For this review, take the finished solid that the model builds, in its own axes (mm). Face numbers are marked on the shaded views. A direction names the side the tool comes from. Coordinates: 2 decimals unless noted, no trailing zeros. Write each loop counter-clockwise with the first axis right and the second up, starting at its lowest first coordinate (ties: lowest second). Pieces come first, ordered by that corner, then holes.
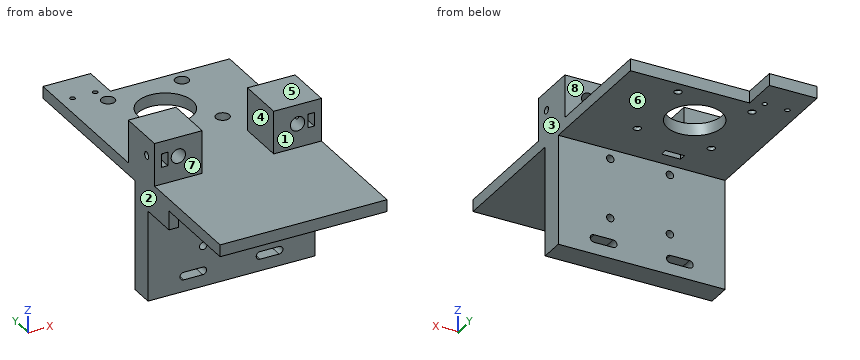
```python
from build123d import *

# Parameters (mm, degrees)
SKETCH1_W           = 70
SKETCH1_H           = 120
BOSS_EXTRUDE1_DEPTH = 5
SKETCH2_W           = 20
SKETCH2_H           = 20
BOSS_EXTRUDE2_DEPTH = 18
CUT_EXTRUDE1_REACH  = 83.572
SKETCH3_R           = 3
CUT_EXTRUDE2_REACH  = 75.171
SKETCH4_R           = 11.5
SKETCH4_R_2         = 1.55
SKETCH5_W           = 20
SKETCH5_H           = 15
SKETCH5_R           = 1.05
BOSS_EXTRUDE3_DEPTH = 5
SKETCH6_W           = 70
SKETCH6_H           = 10
BOSS_EXTRUDE4_DEPTH = 46
SKETCH7_W           = 2.6
SKETCH7_H           = 5.7
CUT_EXTRUDE3_DEPTH  = 10
SKETCH8_R           = 1.5
CUT_EXTRUDE4_DEPTH  = 8
CUT_EXTRUDE5_START  = -8
SKETCH9_R           = 1.5
CUT_EXTRUDE5_DEPTH  = 8
SKETCH10_R          = 2.85
CUT_EXTRUDE6_DEPTH  = 3.5
CUT_EXTRUDE7_REACH  = 92.78
SKETCH11_R          = 1.55
CUT_EXTRUDE8_REACH  = 92.78
SKETCH14_W          = 8
SKETCH14_H          = 16
BOSS_EXTRUDE5_DEPTH = 4
CUT_EXTRUDE9_REACH  = 96.689
SKETCH15_W          = 8
SKETCH15_H          = 3


with BuildPart() as part:
    # Sketch1 → Boss-Extrude1 (new body)
    with BuildSketch(Plane.XY):
        Rectangle(SKETCH1_W, SKETCH1_H)
    extrude(amount=BOSS_EXTRUDE1_DEPTH)

    # Sketch2 → Boss-Extrude2 (add)
    with BuildSketch(Plane.XY.offset(5)):
        with Locations((-25, 0)):
            Rectangle(SKETCH2_W, SKETCH2_H)
        with Locations((25, 0)):
            Rectangle(SKETCH2_W, SKETCH2_H)
    extrude(amount=BOSS_EXTRUDE2_DEPTH)

    # Sketch3 → Cut-Extrude1 (cut, up to next)
    with BuildSketch(Plane(origin=(0, 10, 0), x_dir=(1, 0, 0), z_dir=(0, 1, 0)), mode=Mode.PRIVATE) as cut_extrude1_sk1:
        with Locations(Location((-25, -15, 0), (0, 0, 270))):
            Circle(SKETCH3_R)
    cut_extrude1_tool1 = extrude(cut_extrude1_sk1.sketch, amount=-CUT_EXTRUDE1_REACH, mode=Mode.PRIVATE) & part.part
    # Sketch3 → Cut-Extrude1 (cut, up to next)
    with BuildSketch(Plane(origin=(0, 10, 0), x_dir=(1, 0, 0), z_dir=(0, 1, 0)), mode=Mode.PRIVATE) as cut_extrude1_sk2:
        with Locations(Location((25, -15, 0), (0, 0, 270))):
            Circle(SKETCH3_R)
    cut_extrude1_tool2 = extrude(cut_extrude1_sk2.sketch, amount=-CUT_EXTRUDE1_REACH, mode=Mode.PRIVATE) & part.part
    add(cut_extrude1_tool1.solids().sort_by_distance((-25, 10, 15))[0], mode=Mode.SUBTRACT)
    add(cut_extrude1_tool2.solids().sort_by_distance((25, 10, 15))[0], mode=Mode.SUBTRACT)

    # Sketch4 → Cut-Extrude2 (cut, up to next)
    with BuildSketch(Plane(origin=(0, 0, 0), x_dir=(-1, 0, 0), z_dir=(0, 0, -1)), mode=Mode.PRIVATE) as cut_extrude2_sk1:
        with Locations((3.5, 39)):
            Circle(SKETCH4_R)
    cut_extrude2_tool1 = extrude(cut_extrude2_sk1.sketch, amount=-CUT_EXTRUDE2_REACH, mode=Mode.PRIVATE) & part.part
    # Sketch4 → Cut-Extrude2 (cut, up to next)
    with BuildSketch(Plane(origin=(0, 0, 0), x_dir=(-1, 0, 0), z_dir=(0, 0, -1)), mode=Mode.PRIVATE) as cut_extrude2_sk2:
        with Locations((-12, 54.5)):
            Circle(SKETCH4_R_2)
    cut_extrude2_tool2 = extrude(cut_extrude2_sk2.sketch, amount=-CUT_EXTRUDE2_REACH, mode=Mode.PRIVATE) & part.part
    # Sketch4 → Cut-Extrude2 (cut, up to next)
    with BuildSketch(Plane(origin=(0, 0, 0), x_dir=(-1, 0, 0), z_dir=(0, 0, -1)), mode=Mode.PRIVATE) as cut_extrude2_sk3:
        with Locations((19, 54.5)):
            Circle(SKETCH4_R_2)
    cut_extrude2_tool3 = extrude(cut_extrude2_sk3.sketch, amount=-CUT_EXTRUDE2_REACH, mode=Mode.PRIVATE) & part.part
    # Sketch4 → Cut-Extrude2 (cut, up to next)
    with BuildSketch(Plane(origin=(0, 0, 0), x_dir=(-1, 0, 0), z_dir=(0, 0, -1)), mode=Mode.PRIVATE) as cut_extrude2_sk4:
        with Locations((19, 23.5)):
            Circle(SKETCH4_R_2)
    cut_extrude2_tool4 = extrude(cut_extrude2_sk4.sketch, amount=-CUT_EXTRUDE2_REACH, mode=Mode.PRIVATE) & part.part
    # Sketch4 → Cut-Extrude2 (cut, up to next)
    with BuildSketch(Plane(origin=(0, 0, 0), x_dir=(-1, 0, 0), z_dir=(0, 0, -1)), mode=Mode.PRIVATE) as cut_extrude2_sk5:
        with Locations((-12, 23.5)):
            Circle(SKETCH4_R_2)
    cut_extrude2_tool5 = extrude(cut_extrude2_sk5.sketch, amount=-CUT_EXTRUDE2_REACH, mode=Mode.PRIVATE) & part.part
    add(cut_extrude2_tool1.solids().sort_by_distance((-3.5, 39, 0))[0], mode=Mode.SUBTRACT)
    add(cut_extrude2_tool2.solids().sort_by_distance((12, 54.5, 0))[0], mode=Mode.SUBTRACT)
    add(cut_extrude2_tool3.solids().sort_by_distance((-19, 54.5, 0))[0], mode=Mode.SUBTRACT)
    add(cut_extrude2_tool4.solids().sort_by_distance((-19, 23.5, 0))[0], mode=Mode.SUBTRACT)
    add(cut_extrude2_tool5.solids().sort_by_distance((12, 23.5, 0))[0], mode=Mode.SUBTRACT)

    # Sketch5 → Boss-Extrude3 (add)
    with BuildSketch(Plane(origin=(0, 0, 0), x_dir=(-1, 0, 0), z_dir=(0, 0, -1))):
        with Locations((25, 67.5)):
            Rectangle(SKETCH5_W, SKETCH5_H)
        with Locations((20.25, 62)):
            Circle(SKETCH5_R, mode=Mode.SUBTRACT)
        with Locations((29.75, 62)):
            Circle(SKETCH5_R, mode=Mode.SUBTRACT)
    extrude(amount=-BOSS_EXTRUDE3_DEPTH)

    # Sketch6 → Boss-Extrude4 (add)
    with BuildSketch(Plane(origin=(0, 0, 0), x_dir=(-1, 0, 0), z_dir=(0, 0, -1))):
        Rectangle(SKETCH6_W, SKETCH6_H)
    extrude(amount=BOSS_EXTRUDE4_DEPTH)

    # Sketch7 → Cut-Extrude3 (cut)
    with BuildSketch(Plane(origin=(0, -10, 0), x_dir=(1, 0, 0), z_dir=(0, 1, 0))):
        with Locations((30.7, -15)):
            Rectangle(SKETCH7_W, SKETCH7_H)
        with Locations((-30.7, -15)):
            Rectangle(SKETCH7_W, SKETCH7_H)
    extrude(amount=CUT_EXTRUDE3_DEPTH, mode=Mode.SUBTRACT)

    # Sketch8 → Cut-Extrude4 (cut)
    with BuildSketch(Plane(origin=(35, 0, 0), x_dir=(0, 0, -1), z_dir=(1, 0, 0))):
        with Locations((-15, -4)):
            Circle(SKETCH8_R)
    extrude(amount=-CUT_EXTRUDE4_DEPTH, mode=Mode.SUBTRACT)

    # Sketch9 → Cut-Extrude5 (cut)
    with BuildSketch(Plane.ZY.offset(35).offset(CUT_EXTRUDE5_START)):
        with Locations(Location((15, -4, 0), (0, 0, 180))):
            Circle(SKETCH9_R)
    extrude(amount=CUT_EXTRUDE5_DEPTH, mode=Mode.SUBTRACT)

    # Sketch10 → Cut-Extrude6 (cut)
    with BuildSketch(Plane.XY.offset(5)):
        with Locations((-19, 54.5)):
            Circle(SKETCH10_R)
        with Locations((12, 54.5)):
            Circle(SKETCH10_R)
        with Locations((12, 23.5)):
            Circle(SKETCH10_R)
        with Locations((-19, 23.5)):
            Circle(SKETCH10_R)
    extrude(amount=-CUT_EXTRUDE6_DEPTH, mode=Mode.SUBTRACT)

    # Sketch11 → Cut-Extrude7 (cut, up to next)
    with BuildSketch(Plane(origin=(0, 5, 0), x_dir=(1, 0, 0), z_dir=(0, 1, 0)), mode=Mode.PRIVATE) as cut_extrude7_sk1:
        with Locations(Location((-11.805993826, 29, 0), (0, 0, 270))):
            Circle(SKETCH11_R)
    cut_extrude7_tool1 = extrude(cut_extrude7_sk1.sketch, amount=-CUT_EXTRUDE7_REACH, mode=Mode.PRIVATE) & part.part
    # Sketch11 → Cut-Extrude7 (cut, up to next)
    with BuildSketch(Plane(origin=(0, 5, 0), x_dir=(1, 0, 0), z_dir=(0, 1, 0)), mode=Mode.PRIVATE) as cut_extrude7_sk2:
        with Locations(Location((-11.805993826, 4, 0), (0, 0, 270))):
            Circle(SKETCH11_R)
    cut_extrude7_tool2 = extrude(cut_extrude7_sk2.sketch, amount=-CUT_EXTRUDE7_REACH, mode=Mode.PRIVATE) & part.part
    # Sketch11 → Cut-Extrude7 (cut, up to next)
    with BuildSketch(Plane(origin=(0, 5, 0), x_dir=(1, 0, 0), z_dir=(0, 1, 0)), mode=Mode.PRIVATE) as cut_extrude7_sk3:
        with Locations(Location((13.194006174, 29, 0), (0, 0, 270))):
            Circle(SKETCH11_R)
    cut_extrude7_tool3 = extrude(cut_extrude7_sk3.sketch, amount=-CUT_EXTRUDE7_REACH, mode=Mode.PRIVATE) & part.part
    # Sketch11 → Cut-Extrude7 (cut, up to next)
    with BuildSketch(Plane(origin=(0, 5, 0), x_dir=(1, 0, 0), z_dir=(0, 1, 0)), mode=Mode.PRIVATE) as cut_extrude7_sk4:
        with Locations(Location((13.194006174, 4, 0), (0, 0, 270))):
            Circle(SKETCH11_R)
    cut_extrude7_tool4 = extrude(cut_extrude7_sk4.sketch, amount=-CUT_EXTRUDE7_REACH, mode=Mode.PRIVATE) & part.part
    add(cut_extrude7_tool1.solids().sort_by_distance((-11.805994, 5, -29))[0], mode=Mode.SUBTRACT)
    add(cut_extrude7_tool2.solids().sort_by_distance((-11.805994, 5, -4))[0], mode=Mode.SUBTRACT)
    add(cut_extrude7_tool3.solids().sort_by_distance((13.194006, 5, -29))[0], mode=Mode.SUBTRACT)
    add(cut_extrude7_tool4.solids().sort_by_distance((13.194006, 5, -4))[0], mode=Mode.SUBTRACT)

    # Sketch13 → Cut-Extrude8 (cut, up to next)
    with BuildSketch(Plane(origin=(0, 5, 0), x_dir=(1, 0, 0), z_dir=(0, 1, 0)), mode=Mode.PRIVATE) as cut_extrude8_sk1:
        with BuildLine():
            Line((-20, 41.1), (-12, 41.1))
            ThreePointArc((-12, 41.1), (-10.4, 39.5), (-12, 37.9))
            Line((-12, 37.9), (-20, 37.9))
            ThreePointArc((-20, 37.9), (-21.6, 39.5), (-20, 41.1))
        make_face()
    cut_extrude8_tool1 = extrude(cut_extrude8_sk1.sketch, amount=-CUT_EXTRUDE8_REACH, mode=Mode.PRIVATE) & part.part
    # Sketch13 → Cut-Extrude8 (cut, up to next)
    with BuildSketch(Plane(origin=(0, 5, 0), x_dir=(1, 0, 0), z_dir=(0, 1, 0)), mode=Mode.PRIVATE) as cut_extrude8_sk2:
        with BuildLine():
            Line((20, 41.1), (12, 41.1))
            ThreePointArc((12, 41.1), (10.4, 39.5), (12, 37.9))
            Line((12, 37.9), (20, 37.9))
            ThreePointArc((20, 37.9), (21.6, 39.5), (20, 41.1))
        make_face()
    cut_extrude8_tool2 = extrude(cut_extrude8_sk2.sketch, amount=-CUT_EXTRUDE8_REACH, mode=Mode.PRIVATE) & part.part
    add(cut_extrude8_tool1.solids().sort_by_distance((-16, 5, -39.5))[0], mode=Mode.SUBTRACT)
    add(cut_extrude8_tool2.solids().sort_by_distance((16, 5, -39.5))[0], mode=Mode.SUBTRACT)

    # Sketch14 → Boss-Extrude5 (add)
    with BuildSketch(Plane.ZY.offset(35)):
        with Locations((-4, -13)):
            Rectangle(SKETCH14_W, SKETCH14_H)
    extrude(amount=-BOSS_EXTRUDE5_DEPTH)

    # Sketch15 → Cut-Extrude9 (cut, up to next)
    with BuildSketch(Plane(origin=(0, 0, 0), x_dir=(-1, 0, 0), z_dir=(0, 0, -1)), mode=Mode.PRIVATE) as cut_extrude9_sk1:
        with Locations((9, 12.5)):
            Rectangle(SKETCH15_W, SKETCH15_H)
    cut_extrude9_tool1 = extrude(cut_extrude9_sk1.sketch, amount=-CUT_EXTRUDE9_REACH, mode=Mode.PRIVATE) & part.part
    add(cut_extrude9_tool1.solids().sort_by_distance((-9, 12.5, 0))[0], mode=Mode.SUBTRACT)


solid = part.part
```
1) Tool access review of the marked faces 5, 6, 7 and 8: name each direction out of +Z, -Z, +X, -X, +Y, -Y from which nothing blocks a thin tool from reaching the whole face with its end or side.
2) Clearance check with flat-ended pins moving along their axes: P1, Ø3.5, axis at x = -19, y = 23.5, coming from the +Z side; P2, Ø8, axis at x = 4, z = -20, coming from the -Y side; P3, Ø14.5, axis at x = -22.5, z = 16, coming from the +Y side. State where each tip first meets the part, or that it passes through.
3) Consider section C-C (x = 17.5). Give the boundary of the cut face in (y, z), then the cut area to 3 significant figures.
4) Consider section D-D (z = 9.5). Give the boundary of the cut face in (x, y).
5) Consider section A-A (y = 23.5). Give the boundary of the cut face in (x, z), then the cut area to 3 significant figures.
6) For L1, parallel to Y at x = -19, z = 4.15; L2, parallel to X at y = 5, z = 15; L3, parallel to Z at x = -28.4, y = -4, list the stretches that pass through material, from the lowest coordinate up.
7) The part is to be moulded in two halves that separate along X. For the marked faces 1, 2, 3 and 4, say which applies: pulls with the +X half, pulls with the -X half, needs draft (parallel to the pull), parting line crosses it, or undercut.
8) Consider section B-B (z = -4). Give the boundary of the cut face in (x, y), then the cut area to 3 significant figures.
Results:
1. face 5: +Z, +X, -X, +Y, -Y
1. face 6: -Z, +X, -X, +Y
1. face 7: +Z, +X, -X, -Y
1. face 8: +Z, +X, -X, +Y
2. P1: stops at z = 1.5
2. P2: stops at y = -5
2. P3: stops at y = 10
3. outline: (-60, 0) - (-5, 0) - (-5, -37.9) - (5, -37.9) - (5, 0) - (60, 0) - (60, 5) - (10, 5) - (10, 23) - (-10, 23) - (-10, 5) - (-60, 5) - close; (-5, -46) - (5, -46) - (5, -41.1) - (-5, -41.1) - close
3. area: 1,390 mm2
4. outline: (-35, -10) - (-15, -10) - (-15, 10) - (-35, 10) - close; (15, -10) - (35, -10) - (35, 10) - (15, 10) - close
5. outline: (-35, 0) - (-20.55, 0) - (-20.55, 1.5) - (-21.85, 1.5) - (-21.85, 5) - (-35, 5) - close; (-17.45, 0) - (10.45, 0) - (10.45, 1.5) - (9.15, 1.5) - (9.15, 5) - (-16.15, 5) - (-16.15, 1.5) - (-17.45, 1.5) - close; (13.55, 0) - (35, 0) - (35, 5) - (14.85, 5) - (14.85, 1.5) - (13.55, 1.5) - close
5. area: 301 mm2
6. L1: y = -60 to 20.65, 26.35 to 51.65, 57.35 to 75
6. L2: x = -35 to -28, -22 to -15, 15 to 22, 28 to 35
6. L3: z = -46 to 13.5, 16.5 to 23
7. face 1: needs draft
7. face 2: pulls with the -X half
7. face 3: pulls with the +X half
7. face 4: undercut
8. outline: (-35, -21) - (-31, -21) - (-31, -5) - (-13.36, -5) - (-13.36, 5) - (-35, 5) - close; (-10.26, -5) - (11.64, -5) - (11.64, 5) - (-10.26, 5) - close; (14.74, -5) - (35, -5) - (35, 5) - (14.74, 5) - close
8. area: 702 mm2
